Here's how the part is built. I have some questions about the finished solid (model axes, mm). A direction names the side the tool comes from. Coordinates: 2 decimals unless noted, no trailing zeros. Order: outer loops, then holes, each group sorted by start corner. A loop starts at its lowest first (then second) coordinate and runs counter-clockwise, first axis right, second up. Notation, with made-up numbers: M -28.75,38 L -2.75,38 A20 cw -2.75,61 Z; hole C 49.5,-18 d2. An arc over 180 degrees is marked long. One line per question, with ' | ' between items. Start each with the question number.
```python
from build123d import *

# Parameters (mm, degrees)
F0_W      = 15
F0_H      = 8
F1_DEPTH  = 15
F1_TAPER  = 3
F2_R      = 2.5
F3_DEPTH  = 5
F4_R      = 1
F6_R      = 1.5
F7_DEPTH  = 1.5
F8_R      = 1.5
F9_DEPTH  = 3
F10_R     = 1.5
F11_DEPTH = 3


with BuildPart() as f1:
    # F0 (on Top) → F1 (new body)
    with BuildSketch(Plane.XY):
        Rectangle(F0_W, F0_H)
    extrude(amount=F1_DEPTH, taper=F1_TAPER)

    # F2 (on face) → F3 (join)
    with BuildSketch(Plane.XY.offset(15)):
        Circle(F2_R)
    extrude(amount=F3_DEPTH)

    # F4
    f4_edges = [f1.edges().sort_by_distance(p)[0] for p in [
        (7.106942, -3.606942, 7.5),
        (7.106942, 3.606942, 7.5),
        (0, 3.213883, 15),
        (6.713883, 0, 15),
        (0, -3.213883, 15),
        (-6.713883, 0, 15),
        (-7.106942, -3.606942, 7.5),
        (-7.106942, 3.606942, 7.5),
    ]]
    fillet(f4_edges, radius=F4_R)

    # F6 (on Right) → F7 (join, symmetric)
    with BuildSketch(Plane.YZ):
        with Locations((0, 11.0523359562)):
            Circle(F6_R)
    extrude(amount=F7_DEPTH, both=True)

    # F8 (on face) → F9 (cut)
    with BuildSketch(Plane(origin=(-7.4794571076, 0, 0.3919817373), x_dir=(0, -1, 0), z_dir=(-0.9986295348, 0, 0.0523359562))):
        with Locations((0, 10.6791009514)):
            Circle(F8_R)
    extrude(amount=-F9_DEPTH, mode=Mode.SUBTRACT)

    # F10 (on face) → F11 (cut)
    with BuildSketch(Plane(origin=(7.4794571076, 0, 0.3919817373), x_dir=(0, 1, 0), z_dir=(0.9986295348, 0, 0.0523359562))):
        with Locations((0, 10.6791009514)):
            Circle(F10_R)
    extrude(amount=-F11_DEPTH, mode=Mode.SUBTRACT)


solid = f1.part
```
1. Imagine slicing it at B-B (y = 0). List the corners of the cut face in (x, z) for me, then the cut area to 3 significant figures.
2. Will these pins go through, and if not, where does the flat tip stop? pin 1 (2 mm diameter, centred on y = 0, z = 7, fed in from +X); pin 2 (2.5 mm diameter, centred on x = 4.5, y = -0.5, fed in from +Z); pin 3 (3 mm diameter, centred on x = -1.5, z = 12.5, fed in from +Y).
3. We'd pull the mould along Y, two halves only. Please class faces 1 (the face through (-6.84, 3.33, 7.13)), 2 (the face through (5.51, 0.69, 9.65)), 3 (the face through (0.091, -3.636, 6.947)): released by +Y, released by -Y, zero draft, split by the parting line, or undercut.
4. Which directions (+Z, -Z, +X, -X, +Y, -Y) give clear straight access to the entire face, cutting with the end or side of a thin tool? Please do faces 4 (the face through (-3.44, 2.96, 14.72)), 5 (the face through (-3.38, -2.96, 14.72)), 6 (the face through (-0.54, -2.44, 17.46)).
5. Imagine slicing it at A-A (y = -1.25). List the corners of the cut face in (x, z) for me.
6. I need wall thicknesses on line 1 (Z direction, x = 5, y = 2); line 2 (Y direction, x = -6.5, z = 2.75); line 3 (Z direction, x = 4.5, y = 0). Which ranges of each line are inside material? Lowest first, please.
Entries:
1) outline: M -7.5,0 L 7.5,0 L 7,9.56 L 4,9.4 L 3.85,12.4 L 6.84,12.55 L 6.76,14.05 A1 ccw 5.76,15 L 2.5,15 L 2.5,20 L -2.5,20 L -2.5,15 L -5.76,15 A1 ccw -6.76,14.05 L -6.84,12.55 L -3.85,12.4 L -4,9.4 L -7,9.56 Z | area: 220 mm²
2) pin 1: x = 7.19 | pin 2: z = 15 | pin 3: y = 3.42
3) face 1: released by +Y | face 2: undercut | face 3: released by -Y
4) face 4: +Z, -X, +Y | face 5: +Z, -X, -Y | face 6: +Z
5) outline: M -7.5,0 L 7.5,0 L 6.96,10.23 L 3.97,10.07 L 3.88,11.73 L 6.88,11.88 L 6.76,14.05 A1 ccw 5.76,15 L 2.17,15 L 2.17,20 L -2.17,20 L -2.17,15 L -5.76,15 A1 ccw -6.76,14.05 L -6.88,11.88 L -3.88,11.73 L -3.97,10.07 L -6.96,10.23 Z
6) line 1: 0 to 15 | line 2: -3.85 to 3.85 | line 3: 0 to 9.43, 12.43 to 15
